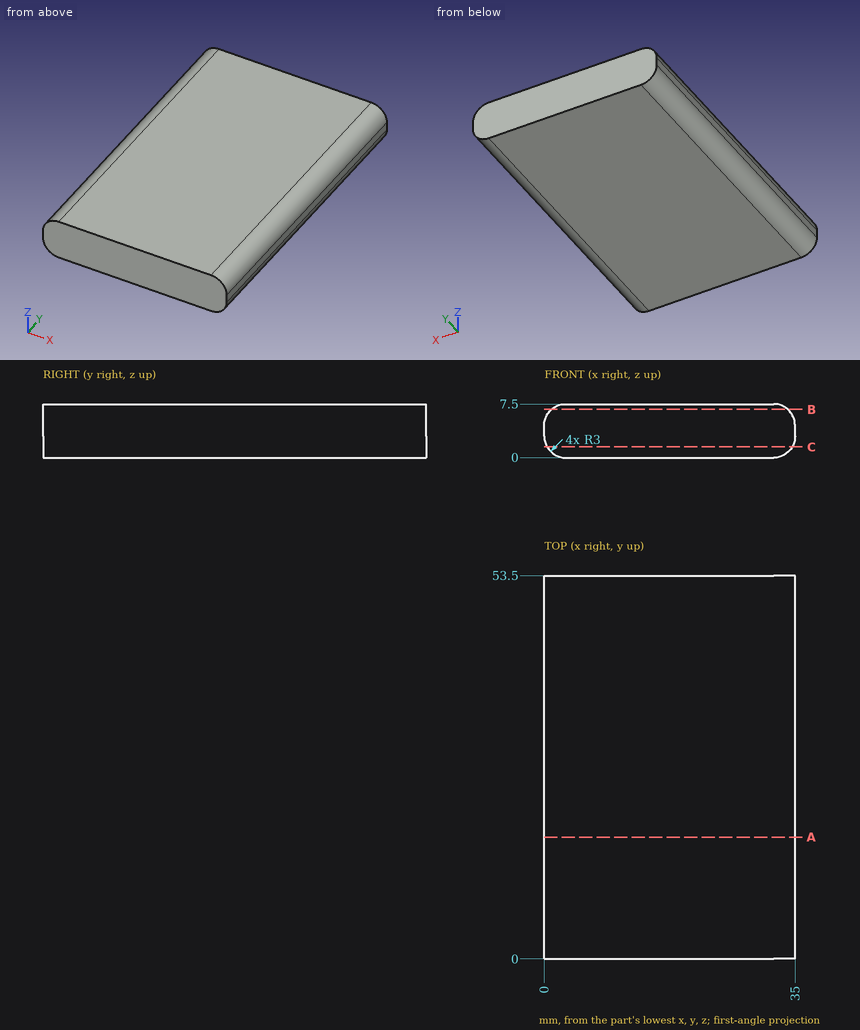
Study the drawing (mm; zero at the part's minimum x, y, z) and answer. Round coordinates to 2 decimals unless told otherwise and drop trailing zeros. Loops run counter-clockwise (first coordinate to the right, second up) from the corner with the lowest first, then second, coordinate; pieces in that order, holes last. Notation, with made-up numbers: (7.5, 54) -> (58.5, 54) arc R10 ccw to (58.5, 60) -> close; hole circle Ø11 at (76, 34.5). An arc over 180 degrees is marked (long way). One line per item, written item: value.
1) A cutting plane is placed at B-B (z = 6.75). Determine the outline of the cut face in (x, y), and give its area (3 significant figures).
Answer list:
outline: (1.02, 0) -> (33.98, 0) -> (33.98, 53.5) -> (1.02, 53.5) -> close
area: 1,760 mm²
2) Consider L1, parallel to X at y = 42.5, z = 4.75; L2, parallel to X at y = 2.5, z = 6. Determine where each line is inside the solid, lowest interval first. Write a range as [from, to].
Answer list:
L1: x = [0.01, 34.99]
L2: x = [0.4, 34.6]
3) A cutting plane is placed at A-A (y = 17). Determine the outline of the cut face in (x, z).
Answer list:
outline: (0, 3) arc R3 ccw to (3, 0) -> (32, 0) arc R3 ccw to (35, 3) -> (35, 4.5) arc R3 ccw to (32, 7.5) -> (3, 7.5) arc R3 ccw to (0, 4.5) -> close
4) A cutting plane is placed at C-C (z = 1.5). Determine the outline of the cut face in (x, y).
Answer list:
outline: (0.4, 0) -> (34.6, 0) -> (34.6, 53.5) -> (0.4, 53.5) -> close
